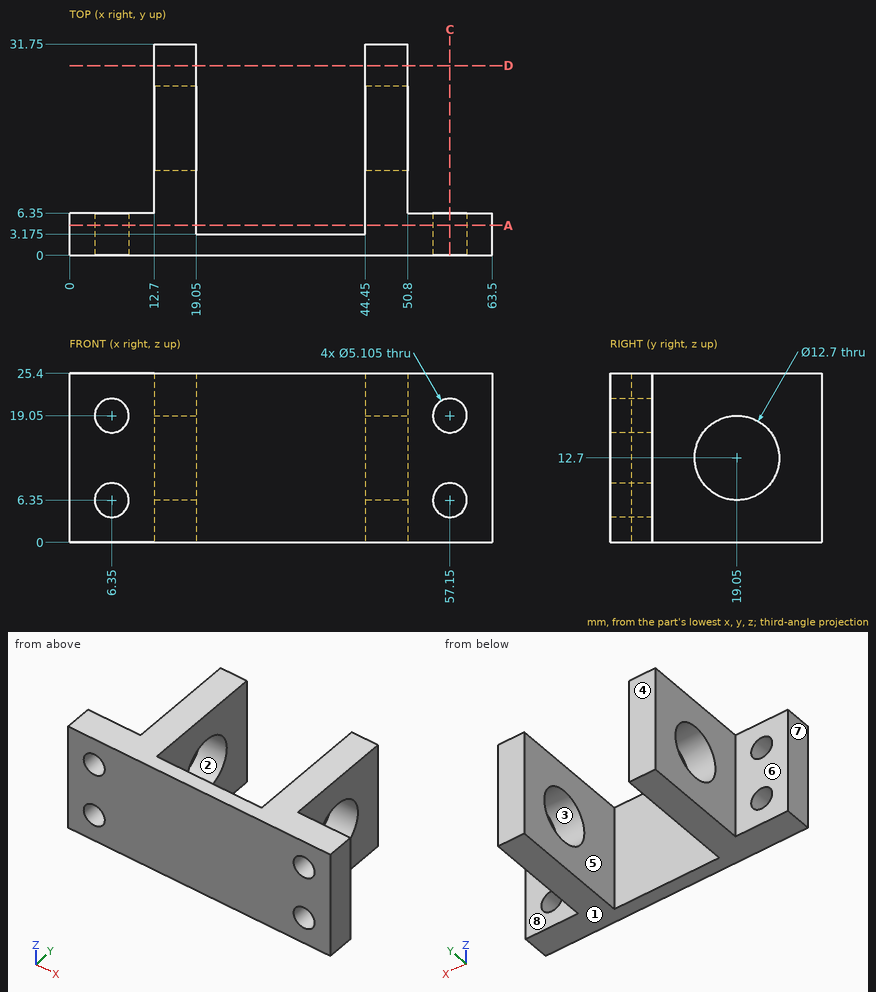
Drawing for the job (mm, zero at the part's lowest x, y, z). A direction names the side the tool comes from. Round coordinates to 2 decimals unless told otherwise and drop trailing zeros. Write each loop counter-clockwise with the first axis right and the second up, starting at its lowest first coordinate (ties: lowest second). Pieces come first, ordered by that corner, then holes. Notation, with made-up numbers: (84, 48) - (94, 48) arc R18 cw to (94, 77) - close; hole circle Ø1 at (13.5, -7). An arc over 180 degrees is marked (long way). Write item = value, one per line. Start each with the question number.
Q1. Which spindle directions (+Z, -Z, +X, -X, +Y, -Y) get a long thin tool onto all of the face, cutting with end or side? Do the marked faces 5, 6, 7 and 8. Say none if no direction does.
Q2. Probe L1, parallel to X at y = 5, z = 6.35; L2, parallel to Z at x = 57.15, y = 3.75; L3, parallel to X at y = 4.5, z = 14.75. List the from-to ranges inside material, lowest first. Write a range as from..to.
Q3. Mould opens along Z. For the marked faces 1, 2, 3 and 4 say: pulls with the +Z half, pulls with the -Z half, needs draft (parallel to the pull), parting line crosses it, or undercut.
Q4. Band-saw the part on A-A (y = 4.5). Count the separate pieces of the cut face and the enclosed holes in it, then the cut area to 3 significant figures.
Q5. Band-saw the part on C-C (x = 57.15). Give the cut face in (y, z).
Q6. Band-saw the part on D-D (y = 28.5). Give the cut face in (x, z).
Q7. Drop flat-ended pins along their axis: pin 1 (12.5 mm diameter, centred on y = 17.5, z = 6.5, fed in from +X); pin 2 (6 mm diameter, centred on x = 6.35, z = 6.35, fed in from +Y); pin 3 (10 mm diameter, centred on y = 13, z = 8, fed in from -X). Give the stop position or say it passes through.
Answers below:
q1.face_5 = +Z, -Z, +Y
q1.face_6 = +Z, -Z, -X, +Y
q1.face_7 = +Z, -Z, -X, +Y, -Y
q1.face_8 = +Z, -Z, +X, +Y
q2.L1 = 0..3.8, 8.9..19.05, 44.45..54.6, 59.7..63.5
q2.L2 = 0..3.8, 8.9..16.5, 21.6..25.4
q2.L3 = 0..19.05, 44.45..63.5
q3.face_1 = pulls with the -Z half
q3.face_2 = undercut
q3.face_3 = undercut
q3.face_4 = needs draft
q4.separate_pieces = 2
q4.enclosed_holes = 4
q4.area = 886 mm2
q5.outline = (0, 0) - (6.35, 0) - (6.35, 3.8) - (0, 3.8) - close; (0, 8.9) - (6.35, 8.9) - (6.35, 16.5) - (0, 16.5) - close; (0, 21.6) - (6.35, 21.6) - (6.35, 25.4) - (0, 25.4) - close
q6.outline = (12.7, 0) - (19.05, 0) - (19.05, 25.4) - (12.7, 25.4) - close; (44.45, 0) - (50.8, 0) - (50.8, 25.4) - (44.45, 25.4) - close
q7.pin_1 = 50.8
q7.pin_2 = 6.35
q7.pin_3 = 12.7
